from build123d import *

# Parameters (mm, degrees)
F0_R     = 9.473878
F1_DEPTH = 12.7
F2_T     = -1.27


with BuildPart() as f1:
    # F0 (on Top) → F1 (new body)
    with BuildSketch(Plane.XY):
        with BuildLine():
            Line((-11.28285, 17.605154), (-11.28285, 0))
            ThreePointArc((-11.28285, 0), (0, -11.28285), (11.28285, 0))
            Line((11.28285, 0), (14.906, 14.071738))
            Line((14.906, 14.071738), (12.07074, 21.969963))
            Line((12.07074, 21.969963), (-7.333735, 21.969963))
            Line((-7.333735, 21.969963), (-11.28285, 17.605154))
        make_face()
        Circle(F0_R, mode=Mode.SUBTRACT)
    extrude(amount=F1_DEPTH)

    # F2
    f2_openings = [f1.faces().sort_by_distance(p)[0] for p in [
        (1.389795, 10.824441, 12.7),
    ]]
    offset(amount=F2_T, openings=f2_openings)


solid = f1.part
Design review of the part built by this model. Coordinates are the model's own, in mm. A direction names the side the tool comes from. Give positions to 0.01 mm unless a question says otherwise; leave off trailing zeros. Loops run counter-clockwise (first coordinate to the right, second up) from the corner with the lowest first, then second, coordinate; pieces in that order, holes last. Notation, with made-up numbers: M 17,7.5 L 27,7.5 A25 cw 27,36.5 Z; hole C 64,58.5 d7. An arc over 180 degrees is marked long. One line per question, with ' | ' between items. Start each with the question number.
1. Add section C-C (z = 3.5). Write out the cut boundary in (x, y).
2. Add section D-D (y = -2.5). Write out the cut boundary in (x, z), plus the area to 3 significant figures.
3. To check wall thickness, follow L1, parallel to Y at x = 0, z = 7.5; L2, parallel to Y at x = 5, z = 11.75; L3, parallel to Z at x = 8, y = 10. State the ranges of each line that lie inside material, in increasing order.
4. For faces 5 (the face through (2, 13, 0)), 6 (the face through (-10.013, 11, 7)), list the 3-axis set-ups (+Z, -Z, +X, -X, +Y, -Y) from which the entire face can be reached by the end or side of a thin tool; tool diameter is ignored.
5. Insertion check: P1, Ø5.5, axis at x = 4.5, z = 9, coming from the -Y side; P2, Ø1, axis at y = 10.5, z = 2.5, coming from the +X side; P3, Ø12, axis at x = -5.5, y = 13.5, coming from the +Z side; P4, Ø9.5, axis at x = 7, y = 15.5, coming from the +Z side. Each pin has a flat end and moves straight along its axis. Give the tip position at first contact, or say it passes through.
6. Add section A-A (x = 0). Write out the cut boundary in (y, z), plus the area to 3 significant figures.
7. The part is to be moulded in two halves that separate along Y. For faces 1 (the face through (13.07, 6.94, 6.26)), 2 (the face through (-9.28, 19.82, 6.26)), 3 (the face through (12.395, 17.308, 6.905)), 4 (the face through (2, 10, 12.7)), say which applies: released by +Y, released by -Y, zero draft, split by the parting line, or undercut.
8. Add section B-B (y = 5). Write out the cut boundary in (x, z), plus the area to 3 significant figures.
Worked out:
1) outline: M -11.28,0 A11.28 ccw 11.28,0 L 14.91,14.07 L 12.07,21.97 L -7.33,21.97 L -11.28,17.61 Z; hole M -10.01,3.9 A10.74 cw 10.53,2.15 L 13.58,14.01 L 11.18,20.7 L -6.77,20.7 L -10.01,17.12 Z; hole C 0,0 d18.95
2) outline: M -11,0 L -9.14,0 L -9.14,12.7 L -11,12.7 Z; M 9.14,0 L 11,0 L 11,12.7 L 9.14,12.7 Z | area: 47.4 mm²
3) L1: y = -11.28 to -9.47, 9.47 to 10.74, 20.7 to 21.97 | L2: y = -10.11 to -8.05, 8.05 to 9.51, 20.7 to 21.97 | L3: z = 0 to 1.27
4) face 5: -Z, +X, -X, +Y, -Y | face 6: +Z
5) P1: stops at y = -11.15 | P2: stops at x = 14.12 | P3: stops at z = 12.7 | P4: stops at z = 1.27
6) outline: M -11.28,0 L -9.47,0 L -9.47,12.7 L -11.28,12.7 Z; M 9.47,0 L 21.97,0 L 21.97,12.7 L 20.7,12.7 L 20.7,1.27 L 10.74,1.27 L 10.74,12.7 L 9.47,12.7 Z | area: 67.9 mm²
7) face 1: released by -Y | face 2: released by +Y | face 3: undercut | face 4: zero draft
8) outline: M -11.28,0 L -8.05,0 L -8.05,12.7 L -9.51,12.7 L -9.51,1.27 L -10.01,1.27 L -10.01,12.7 L -11.28,12.7 Z; M 8.05,0 L 12.57,0 L 12.57,12.7 L 11.26,12.7 L 11.26,1.27 L 9.51,1.27 L 9.51,12.7 L 8.05,12.7 Z | area: 72.8 mm²
